Geometry: final body of the model. Coordinates: model frame, mm. A direction names the side the tool comes from. Round coordinates to 2 decimals unless told otherwise and drop trailing zeros. Loops run counter-clockwise (first coordinate to the right, second up) from the corner with the lowest first, then second, coordinate; pieces in that order, holes last. Notation, with made-up numbers: (-32.5, 52) - (-0.5, 52) arc R7 ccw to (-0.5, 59) - close; hole circle Ø6 at (59.25, 9.5). An arc over 180 degrees is marked (long way). Return JSON: item names as keys, results as strings. Group by question number.
1. Section B-B on z = -3. Count the separate pieces of the cut face and the enclosed holes in it, and give its area (3 significant figures).
2. First-contact query: pin 1 Ø12 at (y, z) = (-9, 18) entering from -X; pin 2 Ø5 at (x, y) = (11.5, -3.5) entering from +Z; pin 3 Ø5 at (x, y) = (35.5, 4) entering from +Z; pin 4 Ø1 at (y, z) = (3.5, 19) entering from +X. Flat tips, straight axial feed; report the tip coordinate or a pass-through.
3. Material intervals for probe 1 along Z at (x, y) = (2.1, 0); probe 2 along Z at (x, y) = (22, 1.25); probe 3 along X at (y, z) = (-7, -24), sorted ascending.
4. Section C-C on y = -8.5. Return loops of the section in (x, z).
5. Section D-D on x = 17. Return loops of the section in (y, z).
6. Section A-A on z = 20. Return loops of the section in (x, y), and give its area (3 significant figures).
7. Draft query along Y for faces 1 (the face through (25.52, 6.74, -0.06)), 2 (the face through (5, -3, -15)), 3 (the face through (3, 9, -29)). Return one class per face: +Y half, -Y half, draft (parallel to the pull), parting line (faces both ways), or undercut.
8. Set-up query: faces 4 (the face through (3, -10, -28)), 5 (the face through (2, 0, 30)), 6 (the face through (3, -3, 19)), 7 (the face through (22, 0, -4)), 8 (the face through (5, -3, 15)). Return all of +Z, -Z, +X, -X, +Y, -Y with unobstructed straight access to the full face (end or side cutting, diameter ignored); none if empty.
from build123d import *

# Parameters (mm, degrees)
F1_W            = 22
F1_H            = 26
F1_H_2          = 8
F2_DEPTH        = 5
F3_DEPTH        = 41
F5_D            = 10.5
F6_D            = 3.2
F7_R            = 10.99999
F8_R            = 5
F10_D           = 5.2
F10_CBORE_D     = 11
F10_CBORE_DEPTH = 2
F11_R           = 5


# Not quite as in the source:
# - a fillet or chamfer is up to 0.001 mm smaller than in the source, because OpenCascade refuses the exact size


with BuildPart() as f2:
    # F1 (on Right) → F2 (new body)
    with BuildSketch(Plane.YZ):
        with Locations((0, 17)):
            Rectangle(F1_W, F1_H)
        Rectangle(F1_W, F1_H_2)
        with Locations((0, -17)):
            Rectangle(F1_W, F1_H)
    extrude(amount=F2_DEPTH)

    # F1 (on Right) → F3 (join)
    with BuildSketch(Plane.YZ):
        Rectangle(F1_W, F1_H_2)
    extrude(amount=F3_DEPTH)

    # F5 (through all)
    with Locations(Plane.XY.offset(4)):
        with Locations((30, 0)):
            Hole(F5_D / 2)

    # F6 (through all)
    with Locations(Plane.XY.offset(4)):
        with Locations((24.3431457505, -5.6568542495), (24.3431457505, 5.6568542495), (35.6568542495, 5.6568542495), (35.6568542495, -5.6568542495)):
            Hole(F6_D / 2)

    # F7 (radius 11 in the source; OpenCascade refuses exactly that, so slightly less here)
    f7_edges = [f2.edges().sort_by_distance(p)[0] for p in [
        (41, 11, 0),
        (41, -11, 0),
    ]]
    fillet(f7_edges, radius=F7_R)

    # F8
    f8_edges = [f2.edges().sort_by_distance(p)[0] for p in [
        (5, 0, 4),
        (5, 0, -4),
    ]]
    fillet(f8_edges, radius=F8_R)

    # F10 (through all)
    with Locations(Plane.YZ.offset(5)):
        with Locations((0, 20), (0, -20)):
            CounterBoreHole(F10_D / 2, F10_CBORE_D / 2, F10_CBORE_DEPTH)

    # F11
    f11_edges = [f2.edges().sort_by_distance(p)[0] for p in [
        (2.5, -11, 30),
        (2.5, 11, 30),
        (2.5, -11, -30),
        (2.5, 11, -30),
    ]]
    fillet(f11_edges, radius=F11_R)


solid = f2.part
Taken from the geometry:
{
 "1": {"separate pieces": "1", "enclosed holes": "5", "area": "731 mm2"},
 "2": {"pin 1": "x = 0", "pin 2": "z = 4.1", "pin 3": "z = 4", "pin 4": "x = 3"},
 "3": {"probe 1": "-30 to -22.6, -17.4 to 17.4, 22.6 to 30", "probe 2": "-4 to 4", "probe 3": "0 to 5"},
 "4": {"outline": "(0, -29.33) - (5, -29.33) - (5, -9) arc R5 cw to (10, -4) - (36.98, -4) - (36.98, 4) - (10, 4) arc R5 cw to (5, 9) - (5, 29.33) - (0, 29.33) - close"},
 "5": {"outline": "(-11, -4) - (11, -4) - (11, 4) - (-11, 4) - close"},
 "6": {"outline": "(0, -11) - (5, -11) - (5, -5.5) - (3, -5.5) - (3, -2.6) - (0, -2.6) - close; (0, 2.6) - (3, 2.6) - (3, 5.5) - (5, 5.5) - (5, 11) - (0, 11) - close", "area": "72.4 mm2"},
 "7": {"face 1": "undercut", "face 2": "draft", "face 3": "+Y half"},
 "8": {"face 4": "-Z, +X, -X, -Y", "face 5": "+Z, +X, -X, +Y, -Y", "face 6": "+X", "face 7": "-Z, +X, +Y, -Y", "face 8": "+Z, +X, +Y, -Y"}
}
